```python
from build123d import *

# Parameters (mm, degrees)
F0_R          = 8.5
F1_DEPTH      = 4
F2_R          = 5
F3_DEPTH      = 100
F5_DEPTH      = 25
F5_DEPTH_BACK = 25
F6_R          = 1.5
F7_DEPTH      = 130.6


with BuildPart() as f1:
    # F0 (on Top) → F1 (new body)
    with BuildSketch(Plane.XY):
        Circle(F0_R)
    extrude(amount=F1_DEPTH)

    # F2 (on Top) → F3 (join)
    with BuildSketch(Plane.XY):
        Circle(F2_R)
    extrude(amount=F3_DEPTH)

    # F4 (on Right) → F5 (cut, two sides)
    with BuildSketch(Plane.YZ) as f5_sk:
        Polygon((0, 101), (-5, 101), (-5, 96), align=None)
    extrude(amount=F5_DEPTH, mode=Mode.SUBTRACT)
    extrude(f5_sk.sketch, amount=-F5_DEPTH_BACK, mode=Mode.SUBTRACT)

    # F6 (on face) → F7 (cut)
    with BuildSketch(Plane(origin=(0, 0, 0), x_dir=(1, 0, 0), z_dir=(0, 0, -1))):
        Circle(F6_R)
    extrude(amount=-F7_DEPTH, mode=Mode.SUBTRACT)


solid = f1.part
```
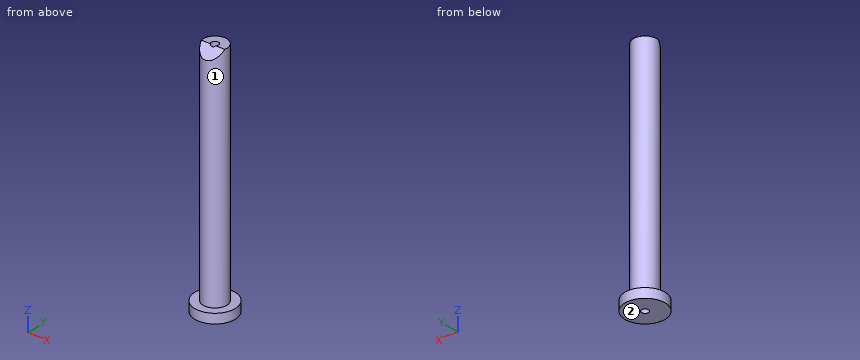
CAD build for the part. Positions are in the model's coordinates, mm. Face numbers are marked on the shaded views. A direction names the side the tool comes from. Round coordinates to 2 decimals unless told otherwise and drop trailing zeros. Write each loop counter-clockwise with the first axis right and the second up, starting at its lowest first coordinate (ties: lowest second). Pieces come first, ordered by that corner, then holes. Notation, with made-up numbers: M 73.25,-31.75 L 95.25,-31.75 A16 cw 95.25,-26.75 Z; hole C 12,76.25 d11. An arc over 180 degrees is marked long. One line per question, with ' | ' between items.
1. Cut at A-A on y = 0. Write the cut outline in (x, z), and give its area (3 significant figures).
Working result:
outline: M -8.5,0 L -1.5,0 L -1.5,100 L -5,100 L -5,4 L -8.5,4 Z; M 1.5,0 L 8.5,0 L 8.5,4 L 5,4 L 5,100 L 1.5,100 Z | area: 728 mm2
2. Probe L1, parallel to Y at x = 0, z = 32.5; L2, parallel to Z at x = -2, y = 5.75. List the from-to ranges inside material, lowest first. Write a range as from..to.
Working result:
L1: -5..-1.5, 1.5..5 | L2: 0..4
3. Pin check, flat tips, straight feed: pin 1 Ø8 at (y, z) = (0.5, 20) entering from +X; pin 2 Ø10 at (x, z) = (5.5, 15.5) entering from -Y; pin 3 Ø1 at (x, y) = (5.5, 1) entering from -Z; pin 4 Ø2 at (y, z) = (3, 15) entering from -X. Stop position of each tip, or through.
Working result:
pin 1: x = 5 | pin 2: y = -4.97 | pin 3: z = 0 | pin 4: x = -4.58
4. Cut at C-C on z = 18. Write the cut outline in (x, y), and give its area (3 significant figures).
Working result:
outline: C 0,0 d10; hole C 0,0 d3 | area: 71.5 mm2
5. Cut at D-D on x = -6.5. Write the cut outline in (y, z), and give its area (3 significant figures).
Working result:
outline: M -5.48,0 L 5.48,0 L 5.48,4 L -5.48,4 Z | area: 43.8 mm2
6. Which spindle directions (+Z, -Z, +X, -X, +Y, -Y) get a long thin tool onto all of the face, cutting with end or side? Do the marked faces 1 and 2. Say none if no direction does.
Working result:
face 1: +Z | face 2: -Z, +X, -X, +Y, -Y
7. Cut at B-B on x = 0. Write the cut outline in (y, z), and give its area (3 significant figures).
Working result:
outline: M -8.5,0 L -1.5,0 L -1.5,99.5 L -5,96 L -5,4 L -8.5,4 Z; M 1.5,0 L 8.5,0 L 8.5,4 L 5,4 L 5,100 L 1.5,100 Z | area: 720 mm2
